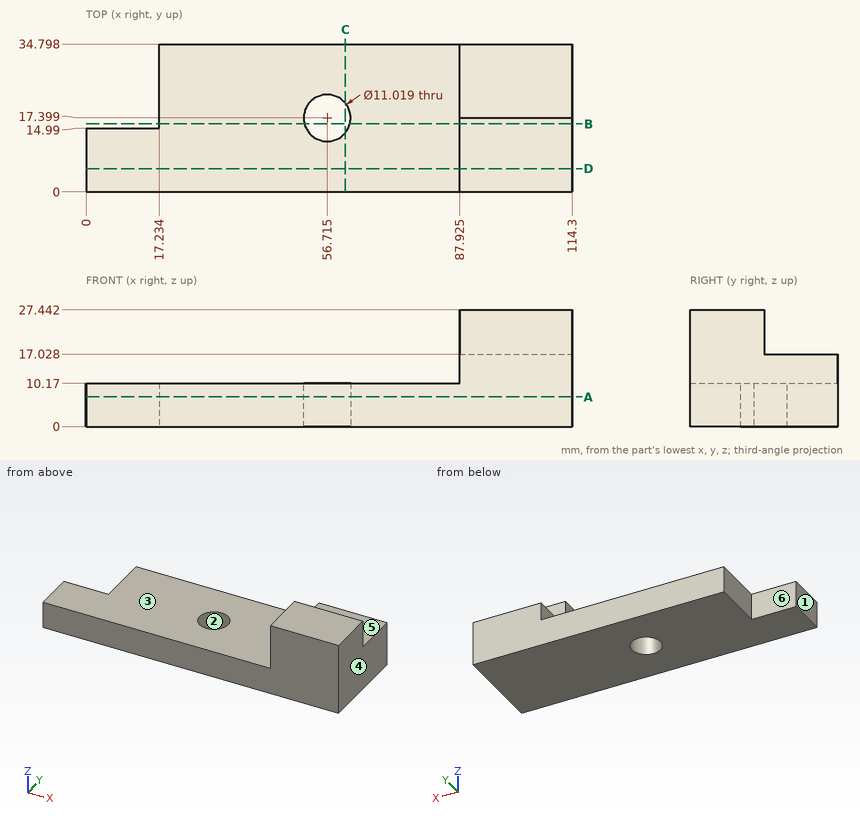
Drawing for the job (mm, zero at the part's lowest x, y, z). A direction names the side the tool comes from. Round coordinates to 2 decimals unless told otherwise and drop trailing zeros. Loops run counter-clockwise (first coordinate to the right, second up) from the corner with the lowest first, then second, coordinate; pieces in that order, holes last. Notation, with made-up numbers: (-17, 11) -> (-6, 11) arc R7 cw to (-6, 16) -> close; hole circle Ø1 at (47, -37.5). An arc over 180 degrees is marked (long way). Answer in a Markdown table with one row per item.
Item 1: Drill centre lines: L1, parallel to X at y = 4, z = 21.5 (1 decimal); L2, parallel to Z at x = 59, y = 4; L3, parallel to X at y = 19.5, z = 7 (1 decimal). Where is each one in solid material? Low to high. Write a range as [from, to].
Answers below:
| item | result |
|---|---|
| L1 | x = [87.9, 114.3] |
| L2 | z = [0, 10.17] |
| L3 | x = [17.2, 51.6], [61.8, 114.3] |
Item 2: Saw through at B-B (y = 16). Write the cut outline in (x, z) (1 decimal), and give its area (3 significant figures).
Answers below:
| item | result |
|---|---|
| outline | (17.2, 0) -> (51.4, 0) -> (51.4, 10.2) -> (17.2, 10.2) -> close; (62, 0) -> (114.3, 0) -> (114.3, 27.4) -> (87.9, 27.4) -> (87.9, 10.2) -> (62, 10.2) -> close |
| area | 1,330 mm² |
Item 3: Saw through at C-C (x = 61). Write the cut outline in (y, z) (1 decimal).
Answers below:
| item | result |
|---|---|
| outline | (0, 0) -> (13.9, 0) -> (13.9, 10.2) -> (0, 10.2) -> close; (20.9, 0) -> (34.8, 0) -> (34.8, 10.2) -> (20.9, 10.2) -> close |
Item 4: Saw through at A-A (z = 7). Write the cut outline in (x, y) (1 decimal), and give its area (3 significant figures).
Answers below:
| item | result |
|---|---|
| outline | (0, 0) -> (114.3, 0) -> (114.3, 34.8) -> (17.2, 34.8) -> (17.2, 15) -> (0, 15) -> close; hole circle Ø11 at (56.7, 17.4) |
| area | 3,540 mm² |
Item 5: Saw through at D-D (y = 5.5). Write the cut outline in (x, z) (1 decimal).
Answers below:
| item | result |
|---|---|
| outline | (0, 0) -> (114.3, 0) -> (114.3, 27.4) -> (87.9, 27.4) -> (87.9, 10.2) -> (0, 10.2) -> close |
Item 6: Mould opens along X. For the marked faces 1, 2 and 3 say: +X half, -X half, draft (parallel to the pull), parting line (faces both ways), or undercut.
Answers below:
| item | result |
|---|---|
| face 1 | -X half |
| face 2 | undercut |
| face 3 | draft |
Item 7: Pin check, flat tips, straight feed: pin 1 (17.5 mm diameter, centred on x = 56.72, y = 17.4, fed in from +Z); pin 2 (11 mm diameter, centred on y = 26.5, z = 7.5, fed in from -X); pin 3 (2 mm diameter, centred on y = 12, z = 15, fed in from -X) (1 decimal). Stop position of each tip, or through.
Answers below:
| item | result |
|---|---|
| pin 1 | stops at z = 10.17 |
| pin 2 | stops at x = 17.23 |
| pin 3 | stops at x = 87.9 |
Item 8: Which spindle directions (+Z, -Z, +X, -X, +Y, -Y) get a long thin tool onto all of the face, cutting with end or side? Do the marked faces 4, 5 and 6. Say none if no direction does.
Answers below:
| item | result |
|---|---|
| face 4 | +Z, -Z, +X, +Y, -Y |
| face 5 | +Z, +X, -X, +Y |
| face 6 | +Z, -Z, -X, +Y |
